The figure shows three views and two pictorial views of one solid part (mm, origin at its lowest corner). Answer the questions. A direction names the side the tool comes from. Coordinates: 2 decimals unless noted, no trailing zeros. Loops run counter-clockwise (first coordinate to the right, second up) from the corner with the lowest first, then second, coordinate; pieces in that order, holes last. Notation, with made-up numbers: M -5,60 L 33,60 A10 ccw 33,75 Z; hole C 3.25,-20.5 d10. An arc over 180 degrees is marked long. Answer as a JSON object with one key per item and string values. Group by question number.
1. A cutting plane is placed at C-C on z = 35. Give the vertices of the cut face in (x, y), and give its area (3 significant figures).
2. For the marked faces 1, 2 and 3, determine the directions among +Z, -Z, +X, -X, +Y, -Y from which every point of the face is accessible in a straight line to the end or side of a thin tool.
3. Determine the mould class of the marked faces 4, 5 and 6 for opening direction X: released by +X, released by -X, zero draft, split by the parting line, or undercut.
4. Given pin 1 (6 mm diameter, centred on y = 69, z = 29, fed in from -X); pin 2 (4 mm diameter, centred on x = 29.5, y = 49, fed in from +Z); pin 3 (12 mm diameter, centred on x = 96.5, z = 65, fed in from +Y), each flat-ended and moving along its own axis, determine where each tip first touches the part or whether it passes through.
5. A cutting plane is placed at D-D on x = 18.5. Give the vertices of the cut face in (y, z).
6. A cutting plane is placed at A-A on z = 24. Give the vertices of the cut face in (x, y), and give its area (4 significant figures).
7. Straight lines are drawn through the part: L1, parallel to Z at x = 58, y = 39; L2, parallel to Y at x = 6, z = 38; L3, parallel to Y at x = 68.5, z = 52. For each, find the intervals that lie inside material, in ascending order.
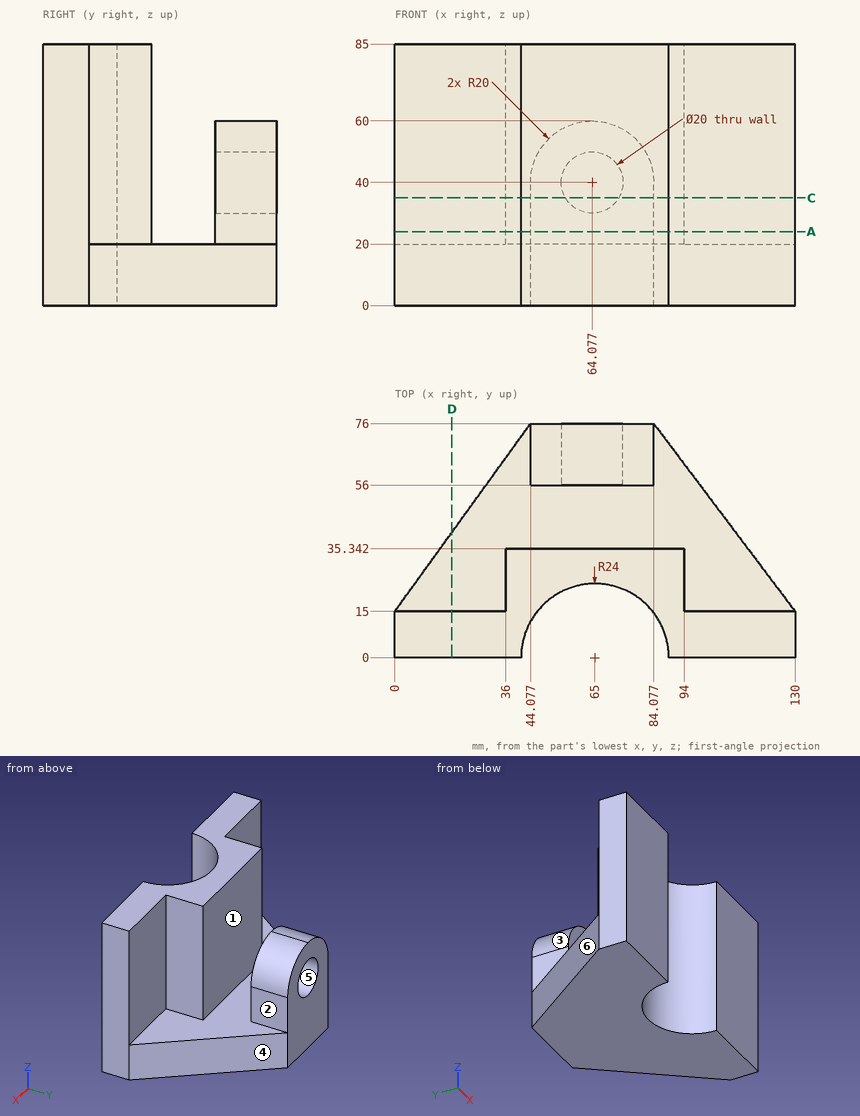
From the geometry:
{
 "1": {"outline": "M 0,0 L 41,0 A24 cw 89,0 L 130,0 L 130,15 L 94,15 L 94,35.34 L 36,35.34 L 36,15 L 0,15 Z; M 44.08,56 L 55.42,56 L 55.42,76 L 44.08,76 Z; M 72.74,56 L 84.08,56 L 84.08,76 L 72.74,76 Z", "area": "2,680 mm²"},
 "2": {"face 1": "+Z, +X, -X", "face 2": "+Z, +X, +Y", "face 3": "+Z, -X, +Y"},
 "3": {"face 4": "released by +X", "face 5": "undercut", "face 6": "released by -X"},
 "4": {"pin 1": "stops at x = 44.08", "pin 2": "stops at z = 20", "pin 3": "stops at y = 35.34"},
 "5": {"outline": "M 0,0 L 40.6,0 L 40.6,20 L 15,20 L 15,85 L 0,85 Z"},
 "6": {"outline": "M 0,0 L 41,0 A24 cw 89,0 L 130,0 L 130,15 L 94,15 L 94,35.34 L 36,35.34 L 36,15 L 0,15 Z; M 44.08,56 L 84.08,56 L 84.08,76 L 44.08,76 Z", "area": "3,025 mm²"},
 "7": {"L1": "z = 0 to 20", "L2": "y = 0 to 15", "L3": "y = 23.74 to 35.34, 56 to 76"}
}
